Study the drawing (mm; zero at the part's minimum x, y, z) and answer. Coordinates: 2 decimals unless noted, no trailing zeros. Write each loop counter-clockwise with the first axis right and the second up, starting at its lowest first coordinate (ties: lowest second). Pieces come first, ordered by that corner, then holes. Notation, with made-up numbers: (-4, 85.25) -> (43, 85.25) arc R19 ccw to (43, 90.25) -> close; hole circle Ø4 at (50, 42.25). An arc over 180 degrees is marked (long way). Write item = value, one per line. Start each with the question number.
1) Section A-A (z = 13.5) is taken. Determine the outline of the cut face in (x, y).
2) Section B-B (x = 40) is taken. Determine the outline of the cut face in (y, z).
3) A flat-ended cylindrical pin translates along its axis: pin 1 Ø3 at (x, z) = (40, 85.5) entering from +Y. Find the tip coordinate at first contact, or state that the pin passes through.
4) Find the intervals of material crossed by line 1 along X through (y, z) = (2, 85.5); line 2 along Z through (x, y) = (40, 1.5); line 3 along Z through (x, y) = (39, 2.45), in increasing order. Write a range as from..to.
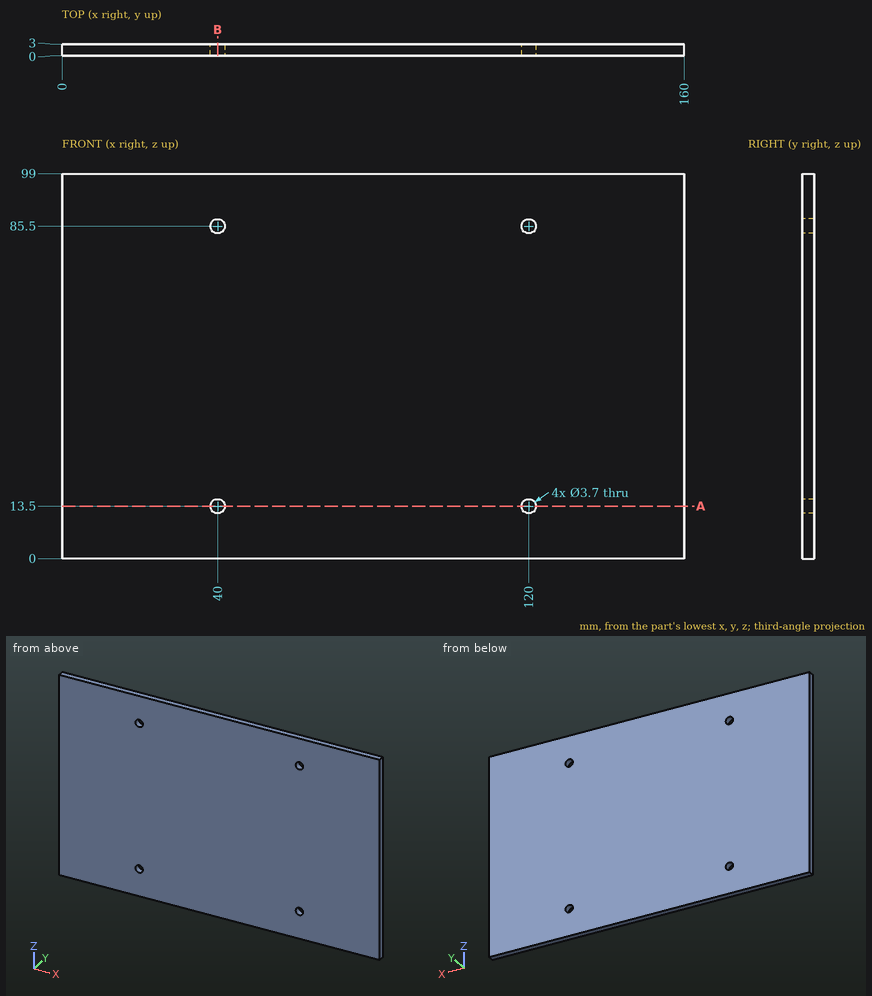
Answer key:
q1.outline = (0, 0) -> (38.15, 0) -> (38.15, 3) -> (0, 3) -> close; (41.85, 0) -> (118.15, 0) -> (118.15, 3) -> (41.85, 3) -> close; (121.85, 0) -> (160, 0) -> (160, 3) -> (121.85, 3) -> close
q2.outline = (0, 0) -> (3, 0) -> (3, 11.65) -> (0, 11.65) -> close; (0, 15.35) -> (3, 15.35) -> (3, 83.65) -> (0, 83.65) -> close; (0, 87.35) -> (3, 87.35) -> (3, 99) -> (0, 99) -> close
q3.pin_1 = through
q4.line_1 = 0..38.15, 41.85..118.15, 121.85..160
q4.line_2 = 0..11.65, 15.35..83.65, 87.35..99
q4.line_3 = 0..11.94, 15.06..83.94, 87.06..99
